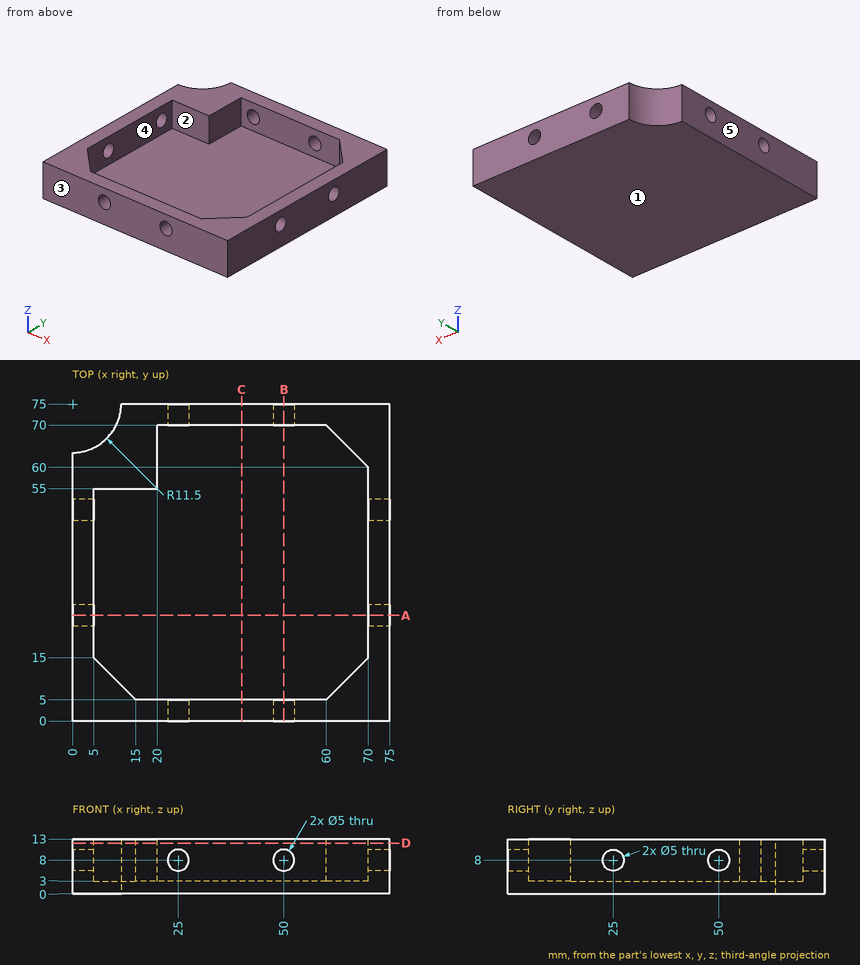
Answer from the drawing. Dimensions are ordinates in mm from the lowest x, y and z of the part. A direction names the side the tool comes from. Coordinates: 2 decimals unless noted, no trailing zeros. Loops run counter-clockwise (first coordinate to the right, second up) from the corner with the lowest first, then second, coordinate; pieces in that order, holes last. Notation, with made-up numbers: (-39, -22) - (19, -22) arc R24 ccw to (19, 0) - close; hole circle Ø5 at (7, 13.25). An arc over 180 degrees is marked (long way). Answer in a Markdown table with one row per item.
1. Which of the six approach directions +Z, -Z, +X, -X, +Y, -Y give full straight-line access (tool end or side, diameter ignored) to the marked faces 4 and 5?
Conclusion:
| item | result |
|---|---|
| face 4 | +Z |
| face 5 | +Z, -Z, -X, +Y, -Y |
2. Find section D-D, the plane z = 12. Write down the section's boundary in (x, y), then the cut area to 3 significant figures.
Conclusion:
| item | result |
|---|---|
| outline | (0, 0) - (75, 0) - (75, 75) - (11.5, 75) arc R11.5 cw to (0, 63.5) - close; hole (5, 15) - (15, 5) - (60, 5) - (70, 15) - (70, 60) - (60, 70) - (20, 70) - (20, 55) - (5, 55) - close |
| area | 1,670 mm² |
3. Find section C-C, the plane x = 40. Write down the section's boundary in (y, z).
Conclusion:
| item | result |
|---|---|
| outline | (0, 0) - (75, 0) - (75, 13) - (70, 13) - (70, 3) - (5, 3) - (5, 13) - (0, 13) - close |
4. Find section A-A, the plane y = 25. Write down the section's boundary in (x, z), then the cut area to 3 significant figures.
Conclusion:
| item | result |
|---|---|
| outline | (0, 0) - (75, 0) - (75, 5.5) - (70, 5.5) - (70, 3) - (5, 3) - (5, 5.5) - (0, 5.5) - close; (0, 10.5) - (5, 10.5) - (5, 13) - (0, 13) - close; (70, 10.5) - (75, 10.5) - (75, 13) - (70, 13) - close |
| area | 275 mm² |
5. Determine the mould class of the marked faces 1, 2 and 3 for opening direction Y: +Y half, -Y half, draft (parallel to the pull), parting line (faces both ways), or undercut.
Conclusion:
| item | result |
|---|---|
| face 1 | draft |
| face 2 | undercut |
| face 3 | -Y half |
6. Straight lines are drawn through the part: line 1 (Z direction, x = 73.2, y = 25); line 2 (X direction, y = 2.95, z = 8); line 3 (Y direction, x = 30, z = 5). For each, find the intervals that lie inside material, in ascending order.
Conclusion:
| item | result |
|---|---|
| line 1 | z = 0 to 5.5, 10.5 to 13 |
| line 2 | x = 0 to 22.5, 27.5 to 47.5, 52.5 to 75 |
| line 3 | y = 0 to 5, 70 to 75 |
7. Given pin 1 (4 mm diameter, centred on x = 25, z = 8, fed in from +Y); pin 2 (2 mm diameter, centred on x = 13, z = 5.5, fed in from -Y); pin 3 (19.5 mm diameter, centred on x = 51.5, y = 45.5, fed in from +Z), each flat-ended and moving along its own axis, determine where each tip first touches the part or whether it passes through.
Conclusion:
| item | result |
|---|---|
| pin 1 | passes through |
| pin 2 | stops at y = 0 |
| pin 3 | stops at z = 3 |
